Build history of the part. All positions in model axes, mm. A direction names the side the tool comes from. Give positions to 0.01 mm unless a question says otherwise; leave off trailing zeros. Write each loop counter-clockwise with the first axis right and the second up, starting at its lowest first coordinate (ties: lowest second). Pieces come first, ordered by that corner, then holes.
from build123d import *

# Parameters (mm, degrees)
SKETCH1_R           = 16.5
BOSS_EXTRUDE1_DEPTH = 50
SKETCH2_R           = 17.5
CUT_EXTRUDE1_DEPTH  = 11
SKETCH3_R           = 2
CUT_EXTRUDE2_DEPTH  = 10


with BuildPart() as part:
    # Sketch1 → Boss-Extrude1 (new body)
    with BuildSketch(Plane.XY):
        with BuildLine():
            Line((-15.968719423, 0), (15.968719423, 0))
            ThreePointArc((15.968719423, 0), (0, 51), (-15.968719423, 0))
        make_face()
        with Locations((0, 23)):
            Circle(SKETCH1_R, mode=Mode.SUBTRACT)
    extrude(amount=BOSS_EXTRUDE1_DEPTH)

    # Sketch2 → Cut-Extrude1 (cut)
    with BuildSketch(Plane.XY.offset(50)):
        with Locations((0, 23)):
            Circle(SKETCH2_R)
    cut_extrude1 = extrude(amount=-CUT_EXTRUDE1_DEPTH, mode=Mode.SUBTRACT)

    # Mirror1: Cut-Extrude1 across plane
    add(cut_extrude1.mirror(Plane.XY.offset(25)), mode=Mode.SUBTRACT)

    # Sketch3 → Cut-Extrude2 (cut)
    with BuildSketch(Plane(origin=(0, 0, 0), x_dir=(-1, 0, 0), z_dir=(0, 0, -1))):
        with Locations((0, 45.5)):
            Circle(SKETCH3_R)
        with Locations((-22.5, 23)):
            Circle(SKETCH3_R)
        with Locations((22.5, 23)):
            Circle(SKETCH3_R)
    cut_extrude2 = extrude(amount=-CUT_EXTRUDE2_DEPTH, mode=Mode.SUBTRACT)

    # Mirror2: Cut-Extrude2 across plane
    add(cut_extrude2.mirror(Plane.XY.offset(25)), mode=Mode.SUBTRACT)


solid = part.part
1. Saw through at C-C on x = -13.5. Give the cut face in (y, z).
2. Drop flat-ended pins along their axis: pin 1 (3 mm diameter, centred on y = 12.5, z = 35, fed in from -X); pin 2 (12 mm diameter, centred on x = 16.5, z = 35.5, fed in from +Y); pin 3 (1.5 mm diameter, centred on x = 16, z = 36, fed in from -Y); pin 4 (1 mm diameter, centred on x = -8.5, y = 35, fed in from +Z). Give the stop position or say it passes through.
3. Mould opens along Y. For faces 1 (the face through (12, 37, 0)), 2 (the face through (23, 23, 10)), 3 (the face through (0.993, 50.982, 24.65)) say: pulls with the +Y half, pulls with the -Y half, needs draft (parallel to the pull), parting line crosses it, or undercut.
4. 3-axis set-ups, long thin cutter, end or side, ignore diameter. For faces 4 (the face through (-22, 23, 10)), 5 (the face through (12, 37, 50)), 6 (the face through (-20.9, 21.8, 45.1)): which of +Z, -Z, +X, -X, +Y, -Y reach the whole face in a straight line?
5. Saw through at D-D on z = 24. Give the cut face in (x, y), plus the area to 3 significant figures.
6. Drill centre lines: line 1 along X through (y, z) = (23.5, 29); line 2 along Y through (x, z) = (0, 21); line 3 along Y through (x, z) = (-10.5, 17). Where is each one in solid material? Low to high.
7. Saw through at B-B on z = 45.5. Give the cut face in (x, y), plus the area to 3 significant figures.
Outcome:
1. outline: (0, 0) - (11.86, 0) - (11.86, 11) - (13.51, 11) - (13.51, 39) - (11.86, 39) - (11.86, 50) - (0, 50) - close; (32.49, 11) - (34.14, 11) - (34.14, 0) - (47.53, 0) - (47.53, 50) - (34.14, 50) - (34.14, 39) - (32.49, 39) - close
2. pin 1: stops at x = -26.51
2. pin 2: stops at y = 48.96
2. pin 3: stops at y = 0
2. pin 4: passes through
3. face 1: needs draft
3. face 2: undercut
3. face 3: parting line crosses it
4. face 4: -Z
4. face 5: +Z, +X, -X, +Y, -Y
4. face 6: +Z
5. outline: (-15.97, 0) - (15.97, 0) arc R28 ccw (long way) to start; hole circle Ø33 at (0, 23)
5. area: 1,500 mm2
6. line 1: x = -28 to -16.49, 16.49 to 28
6. line 2: y = 0 to 6.5, 39.5 to 51
6. line 3: y = 0 to 10.27, 35.73 to 48.96
7. outline: (-15.97, 0) - (15.97, 0) arc R28 ccw (long way) to start; hole circle Ø4 at (-22.5, 23); hole circle Ø35 at (0, 23); hole circle Ø4 at (0, 45.5); hole circle Ø4 at (22.5, 23)
7. area: 1,350 mm2
